from build123d import *

# Parameters (mm, degrees)
F0_W     = 30
F0_H     = 30
F1_DEPTH = 30
F3_R     = 10
F5_DEPTH = 30.001
F4_W     = 20
F4_H     = 20
F6_DEPTH = 30.001
F7_R     = 10
F8_DEPTH = 30.001


with BuildPart() as f1:
    # F0 (on Front) → F1 (new body)
    with BuildSketch(Plane.XZ):
        Rectangle(F0_W, F0_H)
    extrude(amount=F1_DEPTH)

    # F3 (on face) → F5 (cut, through all)
    with BuildSketch(Plane.XZ.offset(30)):
        Circle(F3_R)
    extrude(amount=-F5_DEPTH, mode=Mode.SUBTRACT)

    # F4 (on face) → F6 (cut, through all)
    with BuildSketch(Plane(origin=(-15, 0, 0), x_dir=(0, -1, 0), z_dir=(-1, 0, 0))):
        with Locations((15.342466, 0)):
            Rectangle(F4_W, F4_H)
    extrude(amount=-F6_DEPTH, mode=Mode.SUBTRACT)

    # F7 (on face) → F8 (cut, through all)
    with BuildSketch(Plane.XY.offset(15)):
        with Locations((0, -15)):
            Circle(F7_R)
    extrude(amount=-F8_DEPTH, mode=Mode.SUBTRACT)


solid = f1.part
Here's how the part is built. I have some questions about the finished solid (model axes, mm). A direction names the side the tool comes from. Round coordinates to 2 decimals unless told otherwise and drop trailing zeros. Order: outer loops, then holes, each group sorted by start corner. A loop starts at its lowest first (then second) coordinate and runs counter-clockwise, first axis right, second up. Notation, with made-up numbers: (30.5, 84.25) -> (45.5, 84.25) arc R13 ccw to (45.5, 103.25) -> close; hole circle Ø3 at (51.25, 68.5). An arc over 180 degrees is marked (long way). Return JSON: item names as keys, results as strings.
Q1. If we mould it in two halves opening along Y, with no side actions, what happens to faces 1 (the flat face through (-0.2, 0, 10.2)), 2 (the cylindrical face through (-1.302, -5.085, -12.291)), 3 (the flat face through (15, -14.8, -10.2))? For each: released by +Y, released by -Y, zero draft, split by the parting line, or undercut.
Filled sheet:
{"face 1": "released by +Y", "face 2": "undercut", "face 3": "zero draft"}
Q2. If we section it at C-C on y = -15: List the corners of the cut face in (x, z) for me, plus the area to 3 significant figures.
Filled sheet:
{"outline": "(-15, -15) -> (-10, -15) -> (-10, -10) -> (-15, -10) -> close; (-15, 10) -> (-10, 10) -> (-10, 15) -> (-15, 15) -> close; (10, -15) -> (15, -15) -> (15, -10) -> (10, -10) -> close; (10, 10) -> (15, 10) -> (15, 15) -> (10, 15) -> close", "area": "100 mm^2"}
Q3. Which directions (+Z, -Z, +X, -X, +Y, -Y) give clear straight access to the entire face, cutting with the end or side of a thin tool? Please do faces 4 (the flat face through (11, -25.342, 0)), 5 (the flat face through (-10.2, -14.8, -15)).
Filled sheet:
{"face 4": "+X, -X", "face 5": "-Z, +X, -X, +Y, -Y"}
Q4. If we section it at B-B on z = 0: List the corners of the cut face in (x, y) for me.
Filled sheet:
{"outline": "(-15, -30) -> (-10, -30) -> (-10, -25.34) -> (-15, -25.34) -> close; (-15, -5.34) -> (-10, -5.34) -> (-10, 0) -> (-15, 0) -> close; (10, -30) -> (15, -30) -> (15, -25.34) -> (10, -25.34) -> close; (10, -5.34) -> (15, -5.34) -> (15, 0) -> (10, 0) -> close"}
Q5. For pin 1 Ø10 at (x, y) = (5.5, -18.5) entering from +Z, with a flat end and sliding along its axis, tell me the tip position at first contact or that it passes through.
Filled sheet:
{"pin 1": "stops at z = 15"}
Q6. I need wall thicknesses on line 1 along X through (y, z) = (-15, -12.95); line 2 along Y through (x, z) = (13.25, -5.25). Which ranges of each line are inside material? Lowest first, please. Write a range as from..to.
Filled sheet:
{"line 1": "x = -15..-10, 10..15", "line 2": "y = -30..-25.34, -5.34..0"}
Q7. If we section it at D-D on x = 4.25: List the corners of the cut face in (y, z) for me, plus the area to 3 significant figures.
Filled sheet:
{"outline": "(-30, -15) -> (-24.05, -15) -> (-24.05, -10) -> (-25.34, -10) -> (-25.34, -9.05) -> (-30, -9.05) -> close; (-30, 9.05) -> (-25.34, 9.05) -> (-25.34, 10) -> (-24.05, 10) -> (-24.05, 15) -> (-30, 15) -> close; (-5.95, -15) -> (0, -15) -> (0, -9.05) -> (-5.34, -9.05) -> (-5.34, -10) -> (-5.95, -10) -> close; (-5.95, 10) -> (-5.34, 10) -> (-5.34, 9.05) -> (0, 9.05) -> (0, 15) -> (-5.95, 15) -> close", "area": "138 mm^2"}
Q8. If we section it at A-A on x = -11: List the corners of the cut face in (y, z) for me.
Filled sheet:
{"outline": "(-30, -15) -> (0, -15) -> (0, 15) -> (-30, 15) -> close; hole (-25.34, -10) -> (-5.34, -10) -> (-5.34, 10) -> (-25.34, 10) -> close"}
